Can you work these out from the drawing? Everything is in mm from the part's minimum corner. A direction names the side the tool comes from. Round coordinates to 2 decimals unless told otherwise and drop trailing zeros. Loops run counter-clockwise (first coordinate to the right, second up) from the corner with the lowest first, then second, coordinate; pieces in that order, holes last. Notation, with made-up numbers: M 34.5,76.5 L 55.5,76.5 A31 cw 55.5,110.5 Z; hole C 3.25,45 d7. An arc over 180 degrees is marked long. Return JSON: item names as keys, results as strings. Group by question number.
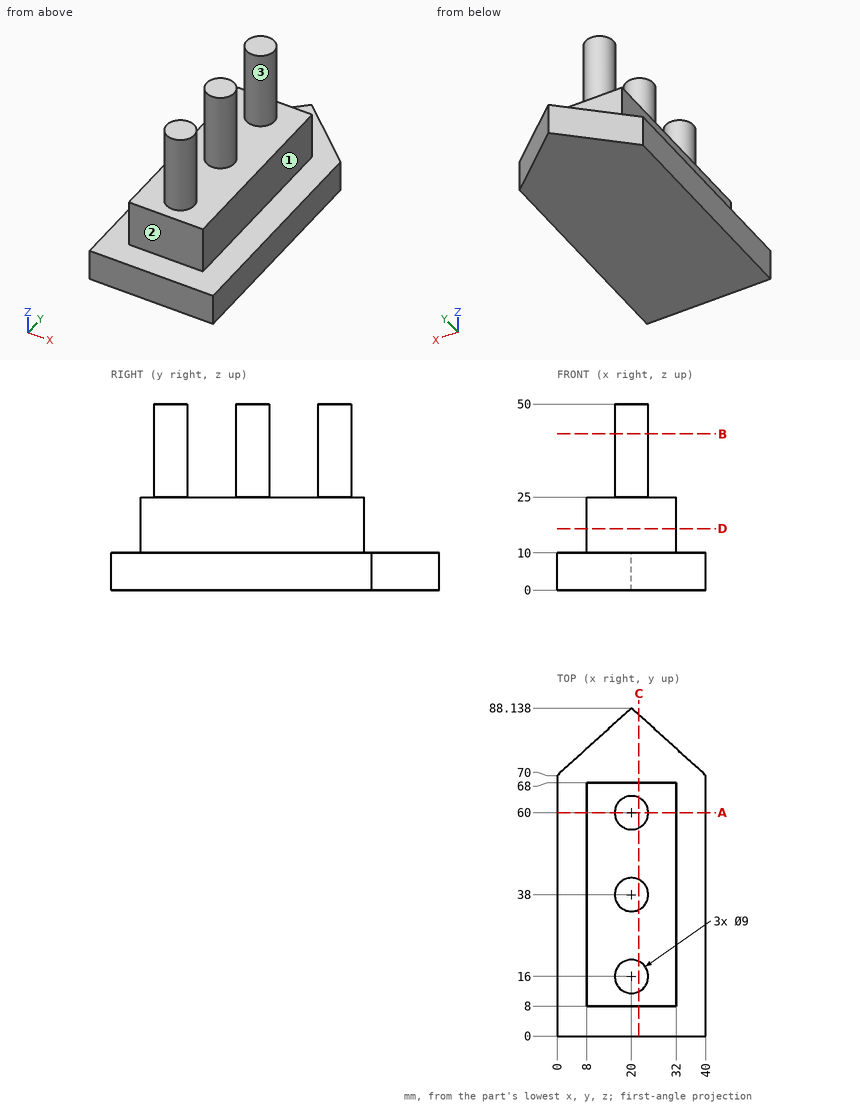
1. If we section it at B-B, the plane z = 42: Please give me the cut outline in (x, y).
2. If we section it at C-C, the plane x = 22: Please give me the cut outline in (y, z) (1 decimal), then the cut area to 3 significant figures.
3. I need wall thicknesses on probe 1 along Z at (x, y) = (22, 21.5); probe 2 along X at (y, z) = (43.5, 17); probe 3 along Z at (x, y) = (37.5, 26). Which ranges of each line are inside material? Lowest first, please.
4. On a 3-axis mill with a long thin cutter (end or side, diameter ignored), from which of +Z, -Z, +X, -X, +Y, -Y can I reach the whole of each face in a straight line? I mean the marked faces 1, 2 and 3. Say none if no direction works.
5. If we section it at A-A, the plane y = 60: Please give me the cut outline in (x, z).
6. I'm going to push flat-ended pins straight in: pin 1 Ø8 at (y, z) = (22, 10.5) entering from -X; pin 2 Ø4.5 at (x, z) = (23.5, 17.5) entering from -Y; pin 3 Ø7 at (x, y) = (25.5, 25.5) entering from +Z; pin 4 Ø16.5 at (y, z) = (32, 20) entering from -X. Where does each tip first touch, or does it pass through?
7. If we section it at D-D, the plane z = 16.5: Please give me the cut outline in (x, y), then the cut area to 3 significant figures.
Geometry results:
{
 "1": {"outline": "C 20,16 d9; C 20,38 d9; C 20,60 d9"},
 "2": {"outline": "M 0,0 L 86.3,0 L 86.3,10 L 68,10 L 68,25 L 64,25 L 64,50 L 56,50 L 56,25 L 42,25 L 42,50 L 34,50 L 34,25 L 20,25 L 20,50 L 12,50 L 12,25 L 8,25 L 8,10 L 0,10 Z", "area": "2,370 mm^2"},
 "3": {"probe 1": "0 to 25", "probe 2": "8 to 32", "probe 3": "0 to 10"},
 "4": {"face 1": "+Z, +X, +Y, -Y", "face 2": "+Z, +X, -X, -Y", "face 3": "+Z"},
 "5": {"outline": "M 0,0 L 40,0 L 40,10 L 32,10 L 32,25 L 24.5,25 L 24.5,50 L 15.5,50 L 15.5,25 L 8,25 L 8,10 L 0,10 Z"},
 "6": {"pin 1": "x = 0", "pin 2": "y = 8", "pin 3": "z = 25", "pin 4": "x = 8"},
 "7": {"outline": "M 8,8 L 32,8 L 32,68 L 8,68 Z", "area": "1,440 mm^2"}
}
